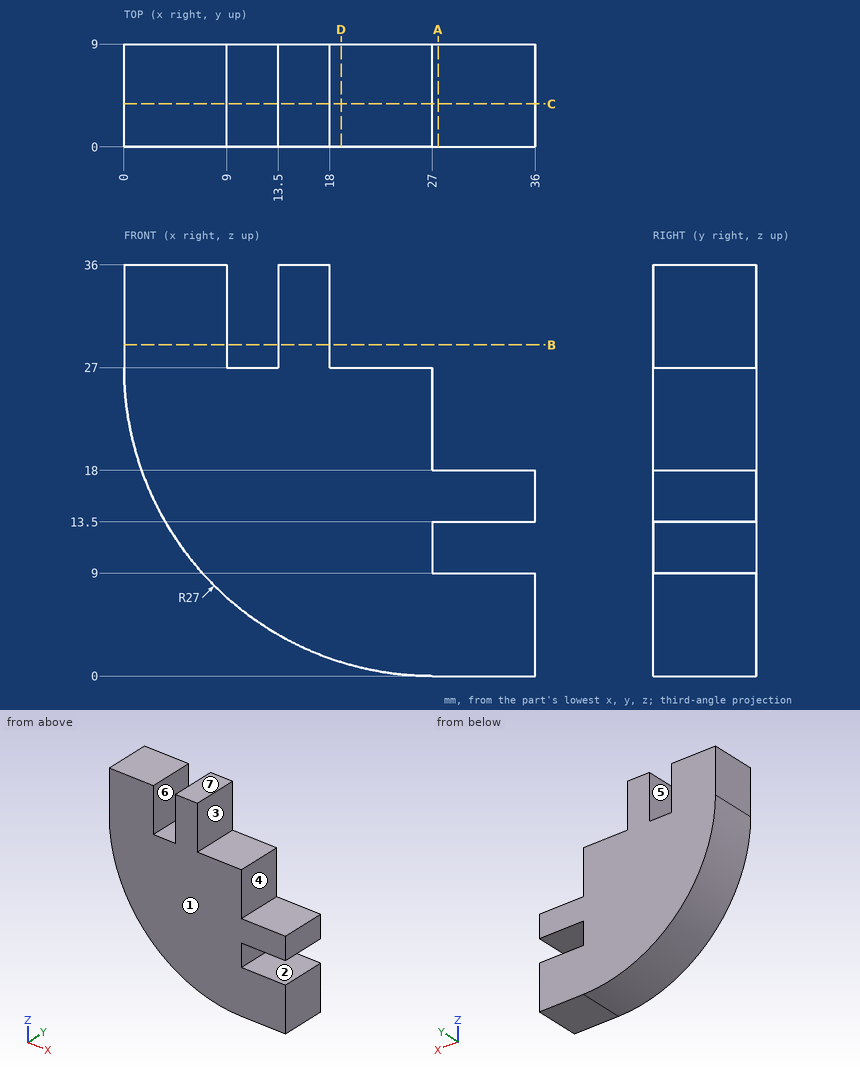
Check sheet for the drawn part. Datum: minimum x, y, z corner. Units: mm. A direction names the side the tool comes from. Round coordinates to 2 decimals unless told otherwise and drop trailing zeros. Loops run counter-clockwise (first coordinate to the right, second up) from the corner with the lowest first, then second, coordinate; pieces in that order, holes last.
Item 1: Gauge pin test, flat ends, axial feed: pin 1 (1 mm diameter, centred on y = 2.5, z = 18, fed in from -X); pin 2 (4.5 mm diameter, centred on y = 6, z = 33, fed in from +X); pin 3 (2 mm diameter, centred on y = 4.5, z = 11.5, fed in from +X). Record the tip position at first contact, or that the pin passes through.
Item 2: Cross-section at D-D on x = 19. Record the boundary of the cut face in (y, z), then the cut area to 3 significant figures.
Item 3: Access from +Z, -Z, +X, -X, +Y, -Y to the whole of each face (thin tool, end or side, straight path). Record for the marked faces 1, 2 and 3.
Item 4: Cross-section at A-A on x = 27.5. Record the boundary of the cut face in (y, z), then the cut area to 4 significant figures.
Item 5: Cross-section at C-C on y = 3.75. Record the boundary of the cut face in (x, z).
Item 6: Cross-section at B-B on z = 29. Record the boundary of the cut face in (x, y).
Item 7: Mould release check, pull along X, two halves, no side actions. Record for the marked faces 4, 5, 6 and 7: pulls with the +X half, pulls with the -X half, needs draft (parallel to the pull), parting line crosses it, or undercut.
Item 8: Thickness scan on line 1 (Z direction, x = 31.5, y = 2); line 2 (X direction, y = 1.75, z = 20); line 3 (X direction, y = 5.25, z = 13). Record the ranges inside material, lowest first.
Answer sheet:
1. pin 1: stops at x = 1.37
1. pin 2: stops at x = 18
1. pin 3: stops at x = 27
2. outline: (0, 1.21) - (9, 1.21) - (9, 27) - (0, 27) - close
2. area: 232 mm2
3. face 1: +Z, -Z, +X, -X, -Y
3. face 2: +X, +Y, -Y
3. face 3: +Z, +X, +Y, -Y
4. outline: (0, 0) - (9, 0) - (9, 9) - (0, 9) - close; (0, 13.5) - (9, 13.5) - (9, 18) - (0, 18) - close
4. area: 121.5 mm2
5. outline: (0, 27) arc R27 ccw to (27, 0) - (36, 0) - (36, 9) - (27, 9) - (27, 13.5) - (36, 13.5) - (36, 18) - (27, 18) - (27, 27) - (18, 27) - (18, 36) - (13.5, 36) - (13.5, 27) - (9, 27) - (9, 36) - (0, 36) - close
6. outline: (0, 0) - (9, 0) - (9, 9) - (0, 9) - close; (13.5, 0) - (18, 0) - (18, 9) - (13.5, 9) - close
7. face 4: pulls with the +X half
7. face 5: undercut
7. face 6: undercut
7. face 7: needs draft
8. line 1: z = 0 to 9, 13.5 to 18
8. line 2: x = 0.92 to 27
8. line 3: x = 3.91 to 27
